Input: dimensioned drawing with shaded views. Units: mm. Origin: part minimum x, y, z. A direction names the side the tool comes from. Give positions to 0.01 mm unless a question says otherwise; leave off trailing zeros. Write each loop counter-clockwise with the first axis right and the second up, starting at its lowest first coordinate (ties: lowest second). Pieces come first, ordered by that corner, then holes.
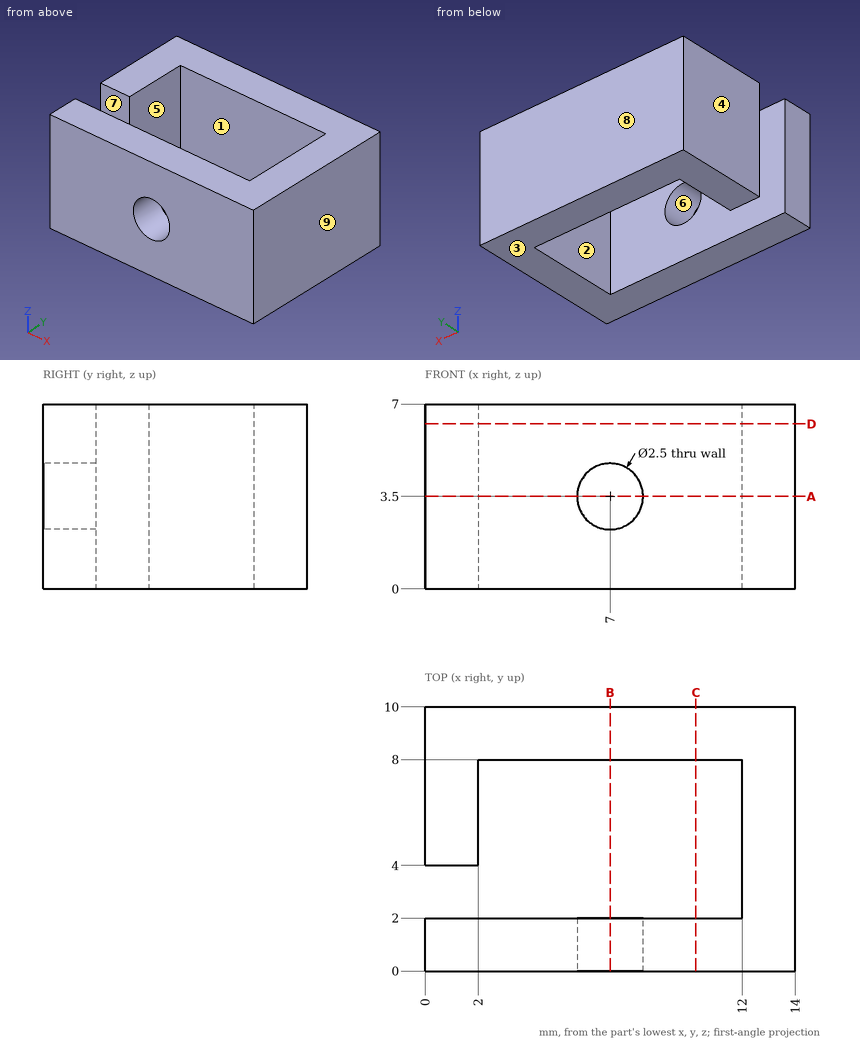
Item 1: Reachability of the marked faces 5, 6, 7, 8 and 9 from +Z, -Z, +X, -X, +Y, -Y: full face, straight path, thin tool, end or side. Return the list, or none.
Found:
face 5: +Z, -Z
face 6: -Y
face 7: +Z, -Z, -X
face 8: +Z, -Z, +X, -X, +Y
face 9: +Z, -Z, +X, +Y, -Y
Item 2: Section A-A, the plane z = 3.5. Return the cut outline in (x, y).
Found:
outline: (0, 0) - (5.75, 0) - (5.75, 2) - (0, 2) - close; (0, 4) - (2, 4) - (2, 8) - (12, 8) - (12, 2) - (8.25, 2) - (8.25, 0) - (14, 0) - (14, 10) - (0, 10) - close
Item 3: Line query: L1, parallel to Y at x = 9, z = 6.75; L2, parallel to X at y = 7, z = 3.75; L3, parallel to Z at x = 7, y = 1.45. Output: solid intervals per line, ascending.
Found:
L1: y = 0 to 2, 8 to 10
L2: x = 0 to 2, 12 to 14
L3: z = 0 to 2.25, 4.75 to 7
Item 4: Pin query (flat end, axial travel): pin 1 Ø4 at (y, z) = (2.5, 1) entering from -X; pin 2 Ø2 at (x, z) = (7, 3.5) entering from -Y. Return the tip coordinate at first contact, or that it passes through.
Found:
pin 1: stops at x = 0
pin 2: stops at y = 8
Item 5: Section D-D, the plane z = 6.25. Return the cut outline in (x, y).
Found:
outline: (0, 0) - (14, 0) - (14, 10) - (0, 10) - (0, 4) - (2, 4) - (2, 8) - (12, 8) - (12, 2) - (0, 2) - close
Item 6: Section C-C, the plane x = 10.25. Return the cut outline in (y, z).
Found:
outline: (0, 0) - (2, 0) - (2, 7) - (0, 7) - close; (8, 0) - (10, 0) - (10, 7) - (8, 7) - close
Item 7: Pull-direction query (X, two-part tool) for the marked faces 1, 2, 3 and 4; classes: +X half, -X half, draft (parallel to the pull), parting line (faces both ways), or undercut.
Found:
face 1: undercut
face 2: undercut
face 3: draft
face 4: -X half
Item 8: Section B-B, the plane x = 7. Return the cut outline in (y, z).
Found:
outline: (0, 0) - (2, 0) - (2, 2.25) - (0, 2.25) - close; (0, 4.75) - (2, 4.75) - (2, 7) - (0, 7) - close; (8, 0) - (10, 0) - (10, 7) - (8, 7) - close
